Print and shaded views of the part. All mm, measured from the part's lowest x, y and z. Give positions to 0.01 mm unless a question says otherwise; leave off trailing zeros. Write each loop counter-clockwise with the first axis right and the second up, starting at its lowest first coordinate (ties: lowest second). Pieces come first, ordered by that corner, then holes. Notation, with made-up numbers: (9.5, -34) - (16.5, -34) arc R29 cw to (16.5, -13) - close; hole circle Ø11 at (57, 28). An arc over 180 degrees is marked (long way). Use one line per item in the form item = value. Start each with the question number.
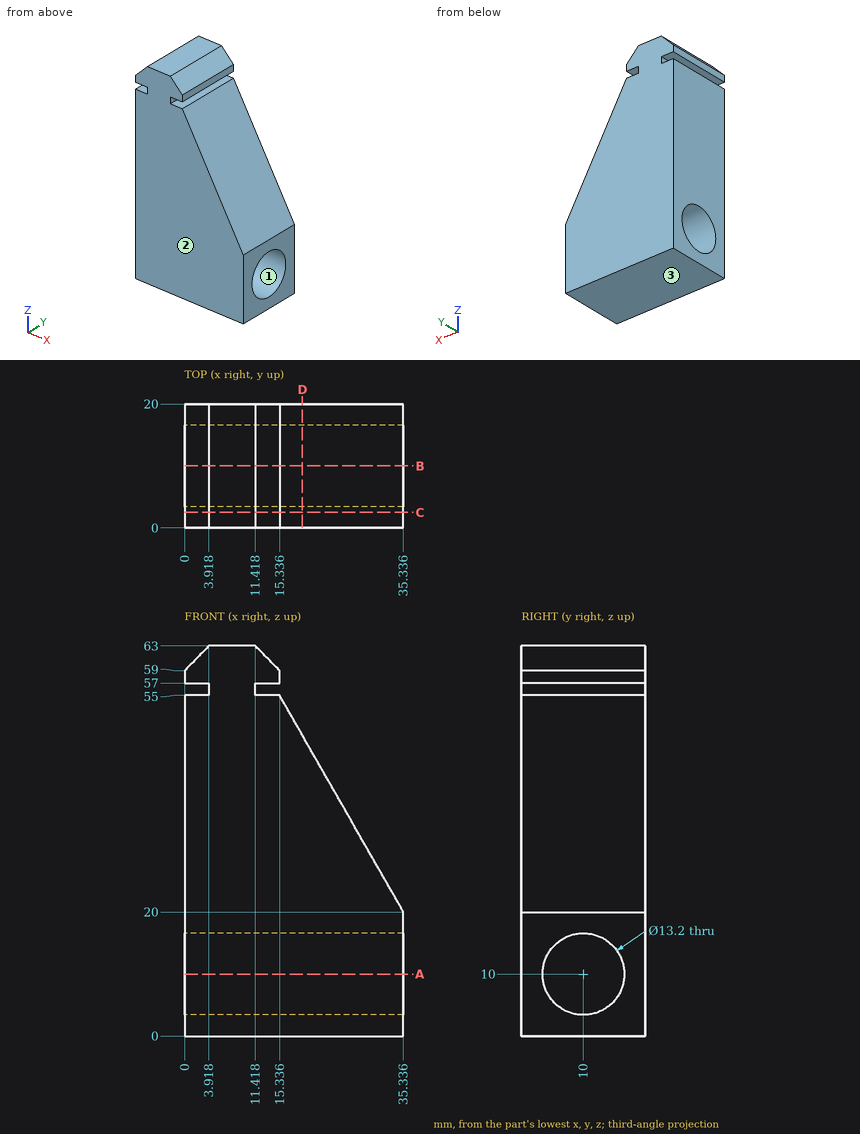
(1) Cut at D-D, the plane x = 19. Give the cut face in (y, z), then the cut area to 3 significant figures.
(2) Pin check, flat tips, straight feed: pin 1 Ø10.5 at (y, z) = (10, 10) entering from -X; pin 2 Ø1.2 at (x, y) = (12.5, 12) entering from +Z; pin 3 Ø0.6 at (y, z) = (7, 56.5) entering from -X; pin 4 Ø1 at (y, z) = (12, 48.5) entering from +X. Stop position of each tip, or through.
(3) Cut at A-A, the plane z = 10. Give the cut face in (x, y), then the cut area to 3 significant figures.
(4) Wall check: line 1 (Z direction, x = 15, y = 10); line 2 (Z direction, x = 12, y = 10) (1 decimal); line 3 (Z direction, x = 24, y = 9) (1 decimal). Give the ranges that are in metal, low to high. Write a range as from..to.
(5) Cut at B-B, the plane y = 10. Give the cut face in (x, z), then the cut area to 3 significant figures.
(6) Cut at C-C, the plane y = 2.5. Give the cut face in (x, z).
(7) Two-plate mould, pull along Y, no slides. Class the marked faces 1, 2 and 3: +Y half, -Y half, draft (parallel to the pull), parting line (faces both ways), or undercut.
Solution:
q1.outline = (0, 0) - (20, 0) - (20, 48.59) - (0, 48.59) - close; hole circle Ø13.2 at (10, 10)
q1.area = 835 mm2
q2.pin_1 = through
q2.pin_2 = 62.51
q2.pin_3 = 3.92
q2.pin_4 = 19.34
q3.outline = (0, 0) - (35.34, 0) - (35.34, 3.4) - (0, 3.4) - close; (0, 16.6) - (35.34, 16.6) - (35.34, 20) - (0, 20) - close
q3.area = 240 mm2
q4.line_1 = 0..3.4, 16.6..55, 57..59.34
q4.line_2 = 0..3.4, 16.6..55, 57..62.4
q4.line_3 = 0..3.5, 16.5..39.8
q5.outline = (0, 0) - (35.34, 0) - (35.34, 3.4) - (0, 3.4) - close; (0, 16.6) - (35.34, 16.6) - (35.34, 20) - (15.34, 55) - (11.42, 55) - (11.42, 57) - (15.34, 57) - (15.34, 59) - (11.42, 63) - (3.92, 63) - (0, 59) - (0, 57) - (3.92, 57) - (3.92, 55) - (0, 55) - close
q5.area = 1,220 mm2
q6.outline = (0, 0) - (35.34, 0) - (35.34, 20) - (15.34, 55) - (11.42, 55) - (11.42, 57) - (15.34, 57) - (15.34, 59) - (11.42, 63) - (3.92, 63) - (0, 59) - (0, 57) - (3.92, 57) - (3.92, 55) - (0, 55) - close
q7.face_1 = undercut
q7.face_2 = -Y half
q7.face_3 = draft
